from build123d import *

# Parameters (mm, degrees)
SKETCH1_W           = 60
SKETCH1_H           = 60
BOSS_EXTRUDE1_DEPTH = 4
SKETCH2_R           = 2.25
CUT_EXTRUDE1_DEPTH  = 4
CUT_EXTRUDE2_DEPTH  = 4


with BuildPart() as part:
    # Sketch1 → Boss-Extrude1 (new body)
    with BuildSketch(Plane.XY):
        Rectangle(SKETCH1_W, SKETCH1_H)
    extrude(amount=BOSS_EXTRUDE1_DEPTH)

    # Sketch2 → Cut-Extrude1 (cut)
    with BuildSketch(Plane.XY.offset(4)):
        with Locations((-25, 25)):
            Circle(SKETCH2_R)
        with Locations((25, 25)):
            Circle(SKETCH2_R)
        with Locations((25, -25)):
            Circle(SKETCH2_R)
        with Locations((-25, -25)):
            Circle(SKETCH2_R)
    extrude(amount=-CUT_EXTRUDE1_DEPTH, mode=Mode.SUBTRACT)

    # Sketch3 → Cut-Extrude2 (cut)
    with BuildSketch(Plane.XY.offset(4)):
        with BuildLine():
            Line((-25, 30), (-30, 30))
            Line((-30, 30), (-30, 25))
            ThreePointArc((-30, 25), (-28.535533906, 28.535533906), (-25, 30))
        make_face()
        with BuildLine():
            ThreePointArc((20.101020514, 26), (21.464466094, 21.464466094), (26, 20.101020514))
            Line((26, 20.101020514), (26, -20.101020514))
            ThreePointArc((26, -20.101020514), (21.464466094, -21.464466094), (20.101020514, -26))
            Line((20.101020514, -26), (-20.101020514, -26))
            ThreePointArc((-20.101020514, -26), (-21.464466094, -21.464466094), (-26, -20.101020514))
            Line((-26, -20.101020514), (-26, 20.101020514))
            ThreePointArc((-26, 20.101020514), (-21.464466094, 21.464466094), (-20.101020514, 26))
            Line((-20.101020514, 26), (20.101020514, 26))
        make_face()
        with BuildLine():
            Line((30, 30), (25, 30))
            ThreePointArc((25, 30), (28.535533906, 28.535533906), (30, 25))
            Line((30, 25), (30, 30))
        make_face()
        with BuildLine():
            ThreePointArc((30, -25), (28.535533906, -28.535533906), (25, -30))
            Line((25, -30), (30, -30))
            Line((30, -30), (30, -25))
        make_face()
        with BuildLine():
            ThreePointArc((-25, -30), (-28.535533906, -28.535533906), (-30, -25))
            Line((-30, -25), (-30, -30))
            Line((-30, -30), (-25, -30))
        make_face()
    extrude(amount=-CUT_EXTRUDE2_DEPTH, mode=Mode.SUBTRACT)


solid = part.part
Design review of the part built by this model. Coordinates are the model's own, in mm. A direction names the side the tool comes from. Coordinates: 2 decimals unless noted, no trailing zeros. Order: outer loops, then holes, each group sorted by start corner. A loop starts at its lowest first (then second) coordinate and runs counter-clockwise, first axis right, second up. Notation, with made-up numbers: M 22,-30.75 L 62,-30.75 A31 cw 62,1.25 Z; hole C 50.5,-38.5 d6. An arc over 180 degrees is marked long. Use a Markdown table: item, result.
(1) Add section A-A (x = -10). Give the boundary of the cut face in (y, z).
Worked answers:
| item | result |
|---|---|
| outline | M -30,0 L -26,0 L -26,4 L -30,4 Z; M 26,0 L 30,0 L 30,4 L 26,4 Z |
(2) For faces 1 (the flat face through (0, 30, 2)), 2 (the flat face through (-26, 0, 2)), list the 3-axis set-ups (+Z, -Z, +X, -X, +Y, -Y) from which the entire face can be reached by the end or side of a thin tool; tool diameter is ignored.
Worked answers:
| item | result |
|---|---|
| face 1 | +Z, -Z, +X, -X, +Y |
| face 2 | +Z, -Z |
(3) Wall thickness on probe 1 along Y at (x, z) = (-25, 2.1); probe 2 along X at (y, z) = (-23, 2); probe 3 along Y at (x, z) = (2.5, 0.3): over which ranges is each line inside the solid? List them lowest first.
Worked answers:
| item | result |
|---|---|
| probe 1 | y = -30 to -27.25, -22.75 to -20, 20 to 22.75, 27.25 to 30 |
| probe 2 | x = -30 to -26.03, -23.97 to -20.42, 20.42 to 23.97, 26.03 to 30 |
| probe 3 | y = -30 to -26, 26 to 30 |
(4) Add section C-C (z = 2). Give the boundary of the cut face in (x, y), then the cut area to 3 significant figures.
Worked answers:
| item | result |
|---|---|
| outline | M -30,-25 A5 ccw -25,-30 L 25,-30 A5 ccw 30,-25 L 30,25 A5 ccw 25,30 L -25,30 A5 ccw -30,25 Z; hole C -25,-25 d4.5; hole C -25,25 d4.5; hole M -26,-20.1 A5 cw -20.1,-26 L 20.1,-26 A5 cw 26,-20.1 L 26,20.1 A5 cw 20.1,26 L -20.1,26 A5 cw -26,20.1 Z; hole C 25,-25 d4.5; hole C 25,25 d4.5 |
| area | 933 mm2 |
(5) Draft analysis for pull direction Y (two halves, no side actions). For faces 3 (the flat face through (0, -30, 2)), 4 (the cylindrical face through (21, 22, 2)), 5 (the flat face through (30, 0, 2)), state which applies: released by +Y, released by -Y, zero draft, split by the parting line, or undercut.
Worked answers:
| item | result |
|---|---|
| face 3 | released by -Y |
| face 4 | undercut |
| face 5 | zero draft |
